```python
from build123d import *

# Parameters (mm, degrees)
ESQUISSE1_W        = 10
ESQUISSE1_H        = 11
ESQUISSE4_R        = 10
BOSS_EXTRU_1_DEPTH = 2
BOSS_EXTRU_1_TAPER = 10
ESQUISSE5_R        = 9.5
BOSS_EXTRU_2_DEPTH = 3
ESQUISSE6_R        = 10
BOSS_EXTRU_3_DEPTH = 9
BOSS_EXTRU_3_DRAFT = -40
CONG_2_R           = 1.5
ESQUISSE7_R        = 7.5
BOSS_EXTRU_4_DEPTH = 7
ESQUISSE8_W        = 2.259893414
ESQUISSE8_H        = 0.706216692
BOSS_EXTRU_5_DEPTH = 7
CONG_3_R           = 1


with BuildPart() as part:
    # Esquisse1 → Révol.-Mince1 (revolve)
    with BuildSketch(Plane(origin=(-11.198304594, 0, 0), x_dir=(1, 0, 0), z_dir=(0, 0, 1)), mode=Mode.PRIVATE) as r_vol_mince1_sk:
        with Locations((5, -13.913919414)):
            Rectangle(ESQUISSE1_W, ESQUISSE1_H)
    revolve(r_vol_mince1_sk.sketch.rotate(Axis((-11.198304594, -8.413919414, 0), (0, -1, 0)), 180), axis=Axis((-11.198304594, -8.413919414, 0), (0, -1, 0)))

    # Esquisse4 → Boss.-Extru.1 (add)
    with BuildSketch(Plane(origin=(0, -8.413919414, 0), x_dir=(1, 0, 0), z_dir=(0, 1, 0))):
        with Locations((-11.245263052, 0)):
            Circle(ESQUISSE4_R)
    extrude(amount=BOSS_EXTRU_1_DEPTH, taper=BOSS_EXTRU_1_TAPER)

    # Esquisse5 → Boss.-Extru.2 (add)
    with BuildSketch(Plane(origin=(0, -6.413919414, 0), x_dir=(1, 0, 0), z_dir=(0, 1, 0))):
        with Locations(Location((-11.36394571, 0, 0), (0, 0, 180))):
            Circle(ESQUISSE5_R)
    extrude(amount=BOSS_EXTRU_2_DEPTH)


with BuildPart() as boss_extru_3_tool:
    # Esquisse6 → Boss.-Extru.3 (with draft: the straight prism first)
    with BuildSketch(Plane(origin=(0, -3.413919414, 0), x_dir=(1, 0, 0), z_dir=(0, 1, 0))):
        with Locations((-11.482628368, 0)):
            Circle(ESQUISSE6_R)
    extrude(amount=BOSS_EXTRU_3_DEPTH)
    # Boss.-Extru.3: the draft: its side faces are tilted about the plane it starts from
    boss_extru_3_sides = [boss_extru_3_tool.faces().sort_by_distance(p)[0] for p in [
        (-21.482628368, 1.086080586, 0),
    ]]
    draft(boss_extru_3_sides, Plane(origin=(0, -3.413919414, 0), x_dir=(1, 0, 0), z_dir=(0, 1, 0)), BOSS_EXTRU_3_DRAFT)


with BuildPart() as part_1:
    add(part.part)

    # Boss.-Extru.3: add boss_extru_3_tool
    add(boss_extru_3_tool.part)

    # Congé2
    cong_2_edges = [part_1.edges().sort_by_distance(p)[0] for p in [
        (-29.034525049, 5.586080586, 0),
        (-1.198304594, -19.413919414, 0),
    ]]
    fillet(cong_2_edges, radius=CONG_2_R)

    # Esquisse7 → Boss.-Extru.4 (add)
    with BuildSketch(Plane(origin=(0, -19.413919414, 0), x_dir=(-1, 0, 0), z_dir=(0, -1, 0))):
        with Locations((11.412006699, 0)):
            Circle(ESQUISSE7_R)
    extrude(amount=BOSS_EXTRU_4_DEPTH)

    # Esquisse8 → Boss.-Extru.5 (add)
    with BuildSketch(Plane(origin=(0, -26.413919414, 0), x_dir=(-1, 0, 0), z_dir=(0, -1, 0))):
        with Locations((14.504595834, -4.896080188)):
            Rectangle(ESQUISSE8_W, ESQUISSE8_H)
        with Locations((8.460660903, -4.896080188)):
            Rectangle(ESQUISSE8_W, ESQUISSE8_H)
        with Locations((11.460660903, -4.896080188)):
            Rectangle(ESQUISSE8_W, ESQUISSE8_H)
    extrude(amount=BOSS_EXTRU_5_DEPTH)

    # Congé3
    cong_3_edges = [part_1.edges().sort_by_distance(p)[0] for p in [
        (-15.634542541, -33.413919414, 4.896080188),
        (-13.374649127, -33.413919414, 4.896080188),
        (-9.59060761, -33.413919414, 4.896080188),
        (-7.330714196, -33.413919414, 4.896080188),
        (-12.59060761, -33.413919414, 4.896080188),
        (-10.330714196, -33.413919414, 4.896080188),
    ]]
    fillet(cong_3_edges, radius=CONG_3_R)


solid = part_1.part
```
Design review of the part built by this model. Coordinates are the model's own, in mm. A direction names the side the tool comes from. Round coordinates to 2 decimals unless told otherwise and drop trailing zeros. Write each loop counter-clockwise with the first axis right and the second up, starting at its lowest first coordinate (ties: lowest second). Pieces come first, ordered by that corner, then holes. Notation, with made-up numbers: (22.5, 69) -> (36.5, 69) arc R20 cw to (36.5, 90) -> close; hole circle Ø3 at (-39, 16). An arc over 180 degrees is marked (long way). Answer in a Markdown table with one row per item.
Q1. To check wall thickness, follow L1, parallel to Y at x = -16.5, z = 6; L2, parallel to Y at x = -9, z = -3; L3, parallel to Z at x = -14.5, y = -31. State the ranges of each line that lie inside material, in increasing order. Write a range as [from, to].
The answers:
| item | result |
|---|---|
| L1 | [-19.41, 5.59] |
| L2 | [-26.41, 5.59] |
| L3 | [4.54, 5.25] |
Q2. Take a section at B-B, the plane y = -13.5. State the section outline as (x, z) points, then the cut area to 3 significant figures.
The answers:
| item | result |
|---|---|
| outline | circle Ø20 at (-11.2, 0) |
| area | 314 mm² |
Q3. Clearance check with flat-ended pins moving along their axes: pin 1 Ø4 at (y, z) = (-14, 8) entering from -X; pin 2 Ø0.7 at (x, y) = (-11.5, -28.5) entering from +Z; pin 3 Ø1.8 at (x, y) = (-15, -28) entering from -Z. State where each tip first meets the part, or that it passes through.
The answers:
| item | result |
|---|---|
| pin 1 | x = -19.2 |
| pin 2 | z = 5.25 |
| pin 3 | z = 4.54 |
Q4. For faces 5 (the face through (-7.616, -33.113, 4.891)), 6 (the face through (-14, -30, 4.543)), 7 (the face through (-11, -30, 5.249)), 8 (the face through (-4, -19.414, -3)), 9 (the face through (-9.31, -33.11, 4.89)), list the 3-axis set-ups (+Z, -Z, +X, -X, +Y, -Y) from which the entire face can be reached by the end or side of a thin tool; tool diameter is ignored.
The answers:
| item | result |
|---|---|
| face 5 | +Z, -Z, +X, -Y |
| face 6 | -Z, +X, -X, -Y |
| face 7 | +Z, +X, -X, -Y |
| face 8 | -Y |
| face 9 | +Z, -Z, -Y |
Q5. Take a section at A-A, the plane y = -5.5. State the section outline as (x, z) points.
The answers:
| item | result |
|---|---|
| outline | circle Ø19 at (-11.36, 0) |
Q6. Draft analysis for pull direction Y (two halves, no side actions). For faces 1 (the face through (-8, -30, 4.543)), 2 (the face through (-13.66, -33.113, 4.891)), 3 (the face through (-19, -3.414, 6)), 4 (the face through (-20.425, -4.935, 2.854)), state which applies: +Y half, -Y half, draft (parallel to the pull), parting line (faces both ways), or undercut.
The answers:
| item | result |
|---|---|
| face 1 | draft |
| face 2 | -Y half |
| face 3 | undercut |
| face 4 | undercut |
